from build123d import *

# Parameters (mm, degrees)
SKETCH1_W            = 21
SKETCH1_H            = 26
SKETCH1_W_2          = 17
SKETCH1_H_2          = 21
BOSS_EXTRUDE1_DEPTH  = 10
SKETCH2_W            = 21
SKETCH2_H            = 26
BOSS_EXTRUDE2_DEPTH  = 2
SKETCH4_W            = 5
SKETCH4_H            = 15
CUT_EXTRUDE2_DEPTH   = 2
SKETCH6_R            = 1.76
BOSS_EXTRUDE3_DEPTH  = 2
SKETCH9_R            = 1.76
BOSS_EXTRUDE5_DEPTH  = 2
SKETCH14_W           = 11
SKETCH14_H           = 1
BOSS_EXTRUDE8_DEPTH  = 8
SKETCH16_R           = 2.1
CUT_EXTRUDE3_DEPTH   = 36
SKETCH17_R           = 1.75
BOSS_EXTRUDE9_DEPTH  = 1.2
SKETCH18_W           = 11
SKETCH18_H           = 14.770488881
CUT_EXTRUDE4_DEPTH   = 3.2
SKETCH19_W           = 11
SKETCH19_H           = 14.236904858
CUT_EXTRUDE5_DEPTH   = 10
SKETCH20_R           = 2.1
BOSS_EXTRUDE10_DEPTH = 1
SKETCH22_W           = 4.498408698
SKETCH22_H           = 14.372964376
CUT_EXTRUDE6_DEPTH   = 10


with BuildPart() as part:
    # Sketch1 → Boss-Extrude1 (new body)
    with BuildSketch(Plane.XY):
        Rectangle(SKETCH1_W, SKETCH1_H)
        Rectangle(SKETCH1_W_2, SKETCH1_H_2, mode=Mode.SUBTRACT)
    extrude(amount=BOSS_EXTRUDE1_DEPTH)

    # Sketch2 → Boss-Extrude2 (add)
    with BuildSketch(Plane.XY.offset(10)):
        Rectangle(SKETCH2_W, SKETCH2_H)
    extrude(amount=BOSS_EXTRUDE2_DEPTH)

    # Sketch4 → Cut-Extrude2 (cut)
    with BuildSketch(Plane(origin=(10.5, 0, 0), x_dir=(0, 0, -1), z_dir=(1, 0, 0))):
        with Locations((-6.8, -2.5)):
            Rectangle(SKETCH4_W, SKETCH4_H)
    extrude(amount=-CUT_EXTRUDE2_DEPTH, mode=Mode.SUBTRACT)

    # Sketch6 → Boss-Extrude3 (add)
    with BuildSketch(Plane.XY.offset(12)):
        with BuildLine():
            Line((0, 13), (5.5, 13))
            Line((5.5, 13), (5.5, 18))
            ThreePointArc((5.5, 18), (0, 23.5), (-5.5, 18))
            Line((-5.5, 18), (-5.5, 13))
            Line((-5.5, 13), (0, 13))
        make_face()
        with Locations((0, 18)):
            Circle(SKETCH6_R, mode=Mode.SUBTRACT)
    extrude(amount=-BOSS_EXTRUDE3_DEPTH)

    # Sketch9 → Boss-Extrude5 (add)
    with BuildSketch(Plane.XY.offset(12)):
        with BuildLine():
            Line((0, -13), (-5.5, -13))
            Line((-5.5, -13), (-5.5, -18))
            ThreePointArc((-5.5, -18), (0, -23.5), (5.5, -18))
            Line((5.5, -18), (5.5, -13))
            Line((5.5, -13), (0, -13))
        make_face()
        with Locations((0, -18)):
            Circle(SKETCH9_R, mode=Mode.SUBTRACT)
    extrude(amount=-BOSS_EXTRUDE5_DEPTH)

    # Sketch14 → Boss-Extrude8 (add)
    with BuildSketch(Plane(origin=(0, 0, 0), x_dir=(-1, 0, 0), z_dir=(0, 0, -1))):
        with Locations((0, -12.5)):
            Rectangle(SKETCH14_W, SKETCH14_H)
        with Locations((0, 12.5)):
            Rectangle(SKETCH14_W, SKETCH14_H)
    extrude(amount=BOSS_EXTRUDE8_DEPTH)

    # Sketch16 → Cut-Extrude3 (cut)
    with BuildSketch(Plane(origin=(0, 13, 0), x_dir=(1, 0, 0), z_dir=(0, 1, 0))):
        with Locations((0, 4)):
            Circle(SKETCH16_R)
    extrude(amount=-CUT_EXTRUDE3_DEPTH, mode=Mode.SUBTRACT)

    # Sketch17 → Boss-Extrude9 (add)
    with BuildSketch(Plane.XY.offset(12)):
        with BuildLine():
            Line((-15.5, -1), (-10.5, -1))
            Line((-10.5, -1), (-10.5, 9))
            Line((-10.5, 9), (-15.5, 9))
            ThreePointArc((-15.5, 9), (-20.5, 4), (-15.5, -1))
        make_face()
        with Locations((-15.5, 4)):
            Circle(SKETCH17_R, mode=Mode.SUBTRACT)
    extrude(amount=-BOSS_EXTRUDE9_DEPTH)

    # Sketch18 → Cut-Extrude4 (cut)
    with BuildSketch(Plane.XY.offset(12)):
        with Locations((0, 20.385244441)):
            Rectangle(SKETCH18_W, SKETCH18_H)
    extrude(amount=-CUT_EXTRUDE4_DEPTH, mode=Mode.SUBTRACT)

    # Sketch19 → Cut-Extrude5 (cut)
    with BuildSketch(Plane.XY.offset(12)):
        with Locations((0, -20.118452429)):
            Rectangle(SKETCH19_W, SKETCH19_H)
    extrude(amount=-CUT_EXTRUDE5_DEPTH, mode=Mode.SUBTRACT)

    # Sketch20 → Boss-Extrude10 (add)
    with BuildSketch(Plane.XZ.offset(13)):
        with BuildLine():
            Line((0, 12), (5.5, 12))
            Line((5.5, 12), (5.5, 20))
            ThreePointArc((5.5, 20), (0, 25.5), (-5.5, 20))
            Line((-5.5, 20), (-5.5, 12))
            Line((-5.5, 12), (0, 12))
        make_face()
        with Locations((0, 20)):
            Circle(SKETCH20_R, mode=Mode.SUBTRACT)
    extrude(amount=-BOSS_EXTRUDE10_DEPTH)

    # Sketch22 → Cut-Extrude6 (cut)
    with BuildSketch(Plane(origin=(0, 0, 10), x_dir=(-1, 0, 0), z_dir=(0, 0, -1))):
        with Locations((5.100019104, 1.989760377)):
            Rectangle(SKETCH22_W, SKETCH22_H)
    extrude(amount=-CUT_EXTRUDE6_DEPTH, mode=Mode.SUBTRACT)


solid = part.part
The listing builds one solid part. Answer for the finished solid, in the listing's coordinates (mm). A direction names the side the tool comes from. Give positions to 0.01 mm unless a question says otherwise; leave off trailing zeros. Order: outer loops, then holes, each group sorted by start corner. A loop starts at its lowest first (then second) coordinate and runs counter-clockwise, first axis right, second up. Notation, with made-up numbers: (6, 0.5) - (14, 0.5) arc R25 ccw to (14, 39.5) - close; hole circle Ø4 at (-25, 40.25). An arc over 180 degrees is marked (long way). Use one line per item in the form item = value.
1) Find section B-B on z = -4. Determine the outline of the cut face in (x, y), and give its area (3 significant figures).
Verdict:
outline = (-5.5, -13) - (-2.1, -13) - (-2.1, -12) - (-5.5, -12) - close; (-5.5, 12) - (-2.1, 12) - (-2.1, 13) - (-5.5, 13) - close; (2.1, -13) - (5.5, -13) - (5.5, -12) - (2.1, -12) - close; (2.1, 12) - (5.5, 12) - (5.5, 13) - (2.1, 13) - close
area = 13.6 mm^2
2) Find section D-D on x = -15. Determine the outline of the cut face in (y, z), and give its area (3 significant figures).
Verdict:
outline = (-1, 10.8) - (2.32, 10.8) - (2.32, 12) - (-1, 12) - close; (5.68, 10.8) - (9, 10.8) - (9, 12) - (5.68, 12) - close
area = 7.98 mm^2
3) The mould has two halves that part along X. Classify faces 1 (the flat face through (-5.5, -12.5, 16.1)), 2 (the flat face through (0, 0, 10)), 3 (the flat face through (10, -3, 4.3)): released by +X, released by -X, zero draft, split by the parting line, or undercut.
Verdict:
face_1 = released by -X
face_2 = undercut
face_3 = zero draft
4) For faces 4 (the flat face through (0, 10.5, 5)), 5 (the flat face through (-13, 9, 11)), 6 (the flat face through (-13, 4, 10.8)), 7 (the flat face through (3, -12, -4)), 8 (the flat face through (5.5, 12.5, -3.9)), determine the directions among +Z, -Z, +X, -X, +Y, -Y from which every point of the face is accessible in a straight line to the end or side of a thin tool.
Verdict:
face_4 = -Z
face_5 = +Z, -Z, -X, +Y
face_6 = -Z, -X, +Y, -Y
face_7 = -Z, +X, -X
face_8 = -Z, +X, +Y, -Y
5) Each of these flat-tipped pins is pushed along its axis until it touches: pin 1 (3 mm diameter, centred on y = -2.5, z = 4.5, fed in from -X); pin 2 (2 mm diameter, centred on x = 9.5, y = -3, fed in from +Z); pin 3 (5 mm diameter, centred on x = 4, z = 22, fed in from +Y); pin 4 (9 mm diameter, centred on x = -1.5, z = 15.5, fed in from +Y). Where does it stop, or does it pass through?
Verdict:
pin_1 = -10.5
pin_2 = 12
pin_3 = -12
pin_4 = 13
6) Find section A-A on x = 0. Determine the outline of the cut face in (y, z), and give its area (3 significant figures).
Verdict:
outline = (-13, -8) - (-12, -8) - (-12, -6.1) - (-13, -6.1) - close; (-13, -1.9) - (-12, -1.9) - (-12, 0) - (-10.5, 0) - (-10.5, 10) - (10.5, 10) - (10.5, 0) - (12, 0) - (12, -1.9) - (13, -1.9) - (13, 12) - (-12, 12) - (-12, 17.9) - (-13, 17.9) - close; (-13, 22.1) - (-12, 22.1) - (-12, 25.5) - (-13, 25.5) - close; (12, -8) - (13, -8) - (13, -6.1) - (12, -6.1) - close
area = 119 mm^2
7) Find section C-C on y = 10. Determine the outline of the cut face in (x, z).
Verdict:
outline = (-10.5, 0) - (-8.5, 0) - (-8.5, 10) - (8.5, 10) - (8.5, 0) - (10.5, 0) - (10.5, 12) - (-10.5, 12) - close
8) Consider probe 1 along Z at (x, y) = (0, -12.25); probe 2 along Y at (x, z) = (-5, -4.5); probe 3 along Y at (x, z) = (-15.5, 11.5). Determine where each line is inside the solid, lowest interval first. Write a range as [from, to].
Verdict:
probe_1 = [-8, -6.1], [-1.9, 17.9], [22.1, 25.5]
probe_2 = [-13, -12], [12, 13]
probe_3 = [-1, 2.25], [5.75, 9]
